Verification items for this drawing (mm, ordinates from the low corner). Coordinates: 2 decimals unless noted, no trailing zeros. Order: outer loops, then holes, each group sorted by start corner. A loop starts at its lowest first (then second) coordinate and runs counter-clockwise, first axis right, second up.
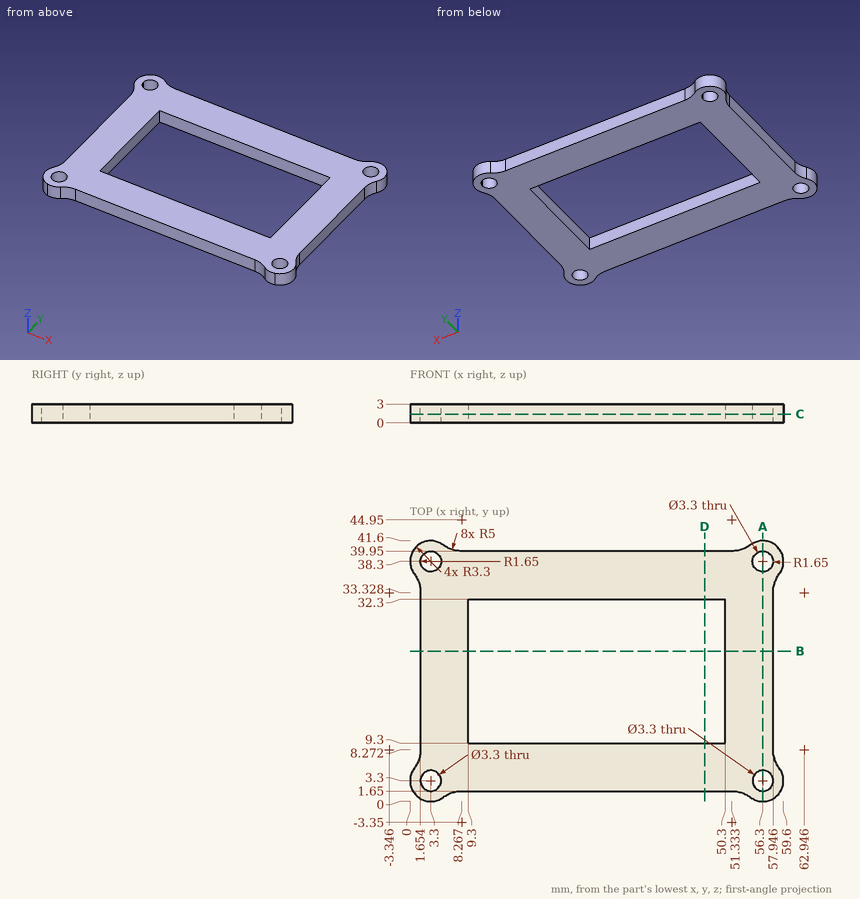
(1) Cross-section at D-D (x = 47). Enter the section's corners in (y, z).
Filled in:
outline: (1.65, 0) - (9.3, 0) - (9.3, 3) - (1.65, 3) - close; (32.3, 0) - (39.95, 0) - (39.95, 3) - (32.3, 3) - close
(2) Cross-section at C-C (z = 1.4). Count the separate pieces of the cut face and the enclosed holes in it, and give its area (3 significant figures).
Filled in:
separate pieces: 1
enclosed holes: 5
area: 1,230 mm2
(3) Cross-section at B-B (y = 24). Enter the section's corners in (x, z).
Filled in:
outline: (1.65, 0) - (9.3, 0) - (9.3, 3) - (1.65, 3) - close; (50.3, 0) - (57.95, 0) - (57.95, 3) - (50.3, 3) - close
(4) Cross-section at A-A (x = 56.3). Enter the section's corners in (y, z), and give its area (3 significant figures).
Filled in:
outline: (0, 0) - (1.65, 0) - (1.65, 3) - (0, 3) - close; (4.95, 0) - (36.65, 0) - (36.65, 3) - (4.95, 3) - close; (39.95, 0) - (41.6, 0) - (41.6, 3) - (39.95, 3) - close
area: 105 mm2
(5) Go/stop test with flat-tipped pins: P1, Ø1.5, axis at x = 34, z = 1.5, coming from the -Y side; P2, Ø3, axis at x = 3.3, y = 3.3, coming from the +Z side; P3, Ø4.5, axis at x = 56.3, y = 3.3, coming from the +Z side; P4, Ø0.9, axis at y = 25.5, z = 2, coming from the +X side. Record where each tip stops, or that it passes through.
Filled in:
P1: stops at y = 1.65
P2: passes through
P3: stops at z = 3
P4: stops at x = 57.95
(6) Thickness scan on probe 1 along Y at (x, z) = (3.3, 0.65); probe 2 along Y at (x, z) = (30, 1.6); probe 3 along X at (y, z) = (28, 2.4). Record the ranges inside material, lowest first.
Filled in:
probe 1: y = 0 to 1.65, 4.95 to 36.65, 39.95 to 41.6
probe 2: y = 1.65 to 9.3, 32.3 to 39.95
probe 3: x = 1.65 to 9.3, 50.3 to 57.95
